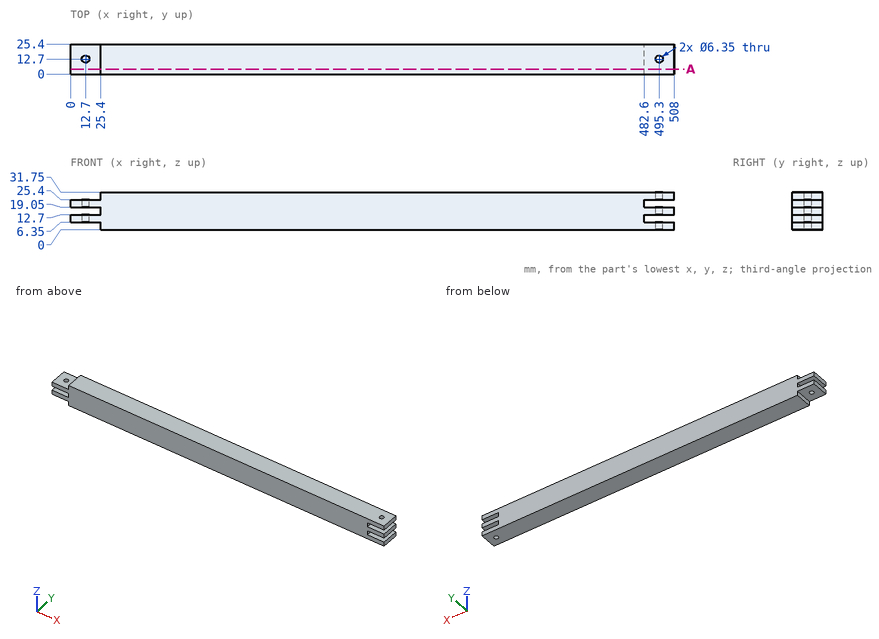
Part print with two shaded views. Sizes in mm from the minimum x, y, z corner. Round coordinates to 2 decimals unless told otherwise and drop trailing zeros. Order: outer loops, then holes, each group sorted by start corner. A loop starts at its lowest first (then second) coordinate and runs counter-clockwise, first axis right, second up. Notation, with made-up numbers: M -17,53.25 L 36,53.25 A16 ccw 36,65.25 Z; hole C 56,-32 d7. An arc over 180 degrees is marked long. Use CSV: the item, a comma, the result in double quotes. Start each with the question number.
(1) Cut at A-A on y = 4.25. List the corners of the cut face in (x, z), then the cut area to 3 significant figures.
(2) Flat gauge pins, fed straight in: P1, Ø5, axis at x = 495.3, y = 12.7, coming from the -Z side; P2, Ø1.5, axis at y = 8, z = 22, coming from the +X side; P3, Ø1.9, axis at y = 7.5, z = 27.5, coming from the -X side; P4, Ø7.5, axis at x = 14.5, y = 8, coming from the -Z side. Where does each tip first touch, or does it go through?
(3) Drill centre lines: probe 1 along X at (y, z) = (12.7, 28.5) (3 decimals); probe 2 along Y at (x, z) = (495.3, 2.5) (3 decimals); probe 3 along X at (y, z) = (12.7, 22.25) (3 decimals). Where is each one in solid material? Low to high.
Findings:
1,outline,"M 0,6.35 L 25.4,6.35 L 25.4,0 L 508,0 L 508,6.35 L 482.6,6.35 L 482.6,12.7 L 508,12.7 L 508,19.05 L 482.6,19.05 L 482.6,25.4 L 508,25.4 L 508,31.75 L 25.4,31.75 L 25.4,25.4 L 0,25.4 L 0,19.05 L 25.4,19.05 L 25.4,12.7 L 0,12.7 Z"
1,area,"15,300 mm^2"
2,P1,"passes through"
2,P2,"stops at x = 482.6"
2,P3,"stops at x = 25.4"
2,P4,"stops at z = 6.35"
3,probe 1,"x = 25.4 to 492.125, 498.475 to 508"
3,probe 2,"y = 0 to 9.525, 15.875 to 25.4"
3,probe 3,"x = 0 to 9.525, 15.875 to 482.6"
